from build123d import *

# Parameters (mm, degrees)
SKETCH_1_R          = 15.9
EXTRUDE_1_DEPTH     = 100
SKETCH_2_W          = 25
SKETCH_2_H          = 15
EXTRUDE_2_DEPTH     = 25
SKETCH_3_R          = 5
CUT_EXTRUDE_1_DEPTH = 129.161499679
SKETCH_4_R          = 14
CUT_EXTRUDE_2_DEPTH = 52


with BuildPart() as part:
    # Эскиз1 → Бобышка-Вытянуть1 (new body)
    with BuildSketch(Plane.XY):
        Circle(SKETCH_1_R)
    extrude(amount=EXTRUDE_1_DEPTH)

    # Эскиз2 → Бобышка-Вытянуть2 (add)
    with BuildSketch(Plane.XY.offset(100)):
        Rectangle(SKETCH_2_W, SKETCH_2_H)
    extrude(amount=EXTRUDE_2_DEPTH)

    # Эскиз3 → Вырез-Вытянуть1 (cut, through all)
    with BuildSketch(Plane(origin=(0, -7.5, 0), x_dir=(1, 0, 0), z_dir=(0, 1, 0))):
        with Locations((0, -112.5)):
            Circle(SKETCH_3_R)
        with BuildLine():
            Line((-12.5, -112.5), (-20.699880193, -112.5))
            Line((-20.699880193, -112.5), (-20.699880193, -150.973701631))
            Line((-20.699880193, -150.973701631), (17.84150118, -150.973701631))
            Line((17.84150118, -150.973701631), (17.84150118, -132.5))
            Line((17.84150118, -132.5), (12.5, -112.5))
            ThreePointArc((12.5, -112.5), (0, -125), (-12.5, -112.5))
        make_face()
    extrude(amount=CUT_EXTRUDE_1_DEPTH, mode=Mode.SUBTRACT)

    # Эскиз4 → Вырез-Вытянуть2 (cut)
    with BuildSketch(Plane(origin=(0, 0, 0), x_dir=(-1, 0, 0), z_dir=(0, 0, -1))):
        Circle(SKETCH_4_R)
    extrude(amount=-CUT_EXTRUDE_2_DEPTH, mode=Mode.SUBTRACT)


solid = part.part
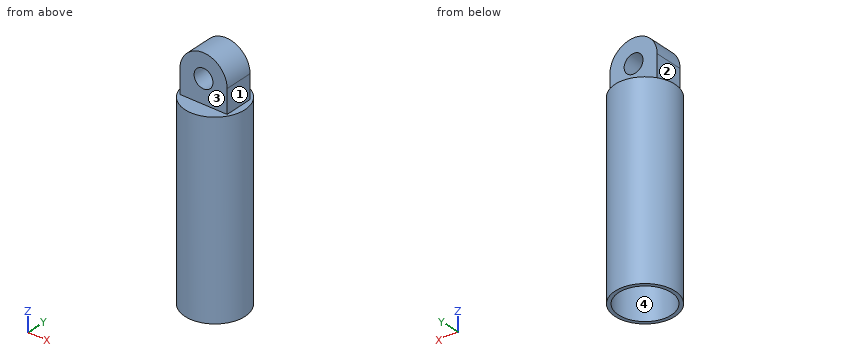
Geometry: final body of the model. Coordinates: model frame, mm. Face numbers are marked on the shaded views. A direction names the side the tool comes from. Round coordinates to 2 decimals unless told otherwise and drop trailing zeros. Loops run counter-clockwise (first coordinate to the right, second up) from the corner with the lowest first, then second, coordinate; pieces in that order, holes last. Notation, with made-up numbers: M 86.5,1 L 129.5,1 A25 ccw 129.5,35 Z; hole C 16.25,-18.5 d8. An arc over 180 degrees is marked long. Put each result on its own line as item: value. Start each with the question number.
(1) Section query C-C (x = 10). Return loops of the section in (y, z), then the cut area to 3 significant figures.
(2) Material intervals for line 1 along X through (y, z) = (-0.75, 112.5); line 2 along Y through (x, z) = (0, 34.5); line 3 along Z through (x, y) = (1, 3.5), sorted ascending. Write a range as [from, to].
(3) Section query A-A (x = 0). Return loops of the section in (y, z).
(4) Section query D-D (z = 35.5). Return loops of the section in (x, y).
(5) Set-up query: the marked faces 1, 2, 3 and 4. Return all of +Z, -Z, +X, -X, +Y, -Y with unobstructed straight access to the full face (end or side cutting, diameter ignored); none if empty.
(6) Section query B-B (y = 2.5). Return loops of the section in (x, z), then the cut area to 3 significant figures.
(7) Contact query for flat-ended pins moving along their axis: pin 1 Ø2 at (x, y) = (-7.5, 6) entering from -Z; pin 2 Ø6 at (y, z) = (2, 104) entering from -X; pin 3 Ø4 at (y, z) = (-2, 107) entering from +X. Output: stop coordinate, or through.
Findings below:
1. outline: M -12.36,0 L -9.8,0 L -9.8,52 L 9.8,52 L 9.8,0 L 12.36,0 L 12.36,100 L 7.5,100 L 7.5,120 L -7.5,120 L -7.5,100 L -12.36,100 Z
1. area: 1,750 mm2
2. line 1: x = [-12.5, -5], [5, 12.5]
2. line 2: y = [-15.9, -14], [14, 15.9]
2. line 3: z = [52, 107.6], [117.4, 124.96]
3. outline: M -15.9,0 L -14,0 L -14,52 L 14,52 L 14,0 L 15.9,0 L 15.9,100 L 7.5,100 L 7.5,107.5 L -7.5,107.5 L -7.5,100 L -15.9,100 Z; M -7.5,117.5 L 7.5,117.5 L 7.5,125 L -7.5,125 Z
4. outline: C 0,0 d31.8; hole C 0,0 d28
5. face 1: +Z, +X, +Y, -Y
5. face 2: +Z, -X, +Y, -Y
5. face 3: +Z, +X, -X, -Y
5. face 4: -Z
6. outline: M -15.7,0 L -13.77,0 L -13.77,52 L 13.77,52 L 13.77,0 L 15.7,0 L 15.7,100 L 12.5,100 L 12.5,112.5 A12.5 ccw -12.5,112.5 L -12.5,100 L -15.7,100 Z; hole C 0,112.5 d10
6. area: 2,190 mm2
7. pin 1: stops at z = 52
7. pin 2: stops at x = -12.5
7. pin 3: stops at x = 12.5
